Could you check a few things on this model? Use its own coordinates, in mm. A direction names the side the tool comes from. Give positions to 0.01 mm unless a question says otherwise; leave off trailing zeros. Order: outer loops, then holes, each group sorted by start corner. A loop starts at its lowest first (then second) coordinate and runs counter-clockwise, first axis right, second up. Notation, with made-up numbers: (80.25, -32) - (111.25, -32) arc R18 cw to (111.25, -16) - close; hole circle Ø6 at (33, 29). An arc over 180 degrees is marked (long way). Put each result on its own line as item: value.
from build123d import *

# Parameters (mm, degrees)
PAD_DEPTH    = 1.5
PAD001_DEPTH = 0.9


with BuildPart() as body:
    # Sketch → Pad (new body)
    with BuildSketch(Plane.XY):
        with BuildLine():
            ThreePointArc((92, 56.2709215446), (72.3076923077, 26.7324600061), (92, -2.8060015324))
            ThreePointArc((91.6153846154, -3.7290784554), (92.2692307692, -3.4598476862), (92, -2.8060015324))
            ThreePointArc((91.6153846154, -3.7290784554), (89, -4.8060015324), (90.0769230769, -7.4213861477))
            ThreePointArc((90.0769230769, -7.4213861477), (95.9615384615, -4.9983092247), (93.5384615385, 0.88630616))
            ThreePointArc((93.5384615385, 52.5786138523), (76.3076923077, 26.7324600061), (93.5384615385, 0.88630616))
            ThreePointArc((93.5384615385, 52.5786138523), (95.9615384615, 58.4632292369), (90.0769230769, 60.88630616))
            ThreePointArc((90.0769230769, 60.88630616), (89, 58.2709215446), (91.6153846154, 57.1939984676))
            ThreePointArc((92, 56.2709215446), (92.2692307692, 56.9247676984), (91.6153846154, 57.1939984676))
        make_face()
    extrude(amount=PAD_DEPTH)

    # Sketch001 → Pad001 (join)
    with BuildSketch(Plane.XY):
        with BuildLine():
            ThreePointArc((0, 20), (29.323857539, 21.0437591192), (58.4992960523, 24.1697536209))
            ThreePointArc((58.4992960523, 24.1697536209), (68.0731220762, 28.4157701053), (74.013620455, 37.0411558783))
            ThreePointArc((74.013620455, 37.0411558783), (74.1652431283, 15.9884962371), (87.3639974769, -0.4136484716))
            ThreePointArc((87.3639974769, -0.4136484716), (75.7108888805, 4.2658460628), (63.1588059736, 4.6370922787))
            ThreePointArc((0, 0), (31.664401924, 1.1608311192), (63.1588059736, 4.6370922787))
            Line((0, 20), (0, 0))
        make_face()
        with BuildLine():
            ThreePointArc((8.0757502279, 6.0764743472), (36.8018825362, 7.5909701802), (65.3605544983, 11.0386695272))
            ThreePointArc((65.3605544983, 11.0386695272), (68.7002124728, 15.6044864983), (64.1343955017, 18.9441444728))
            ThreePointArc((7.9242497721, 14.0750396943), (36.1114820384, 15.5611237014), (64.1343955017, 18.9441444728))
            ThreePointArc((7.9242497721, 14.0750396943), (4.0007173264, 10.0000067928), (8.0757502279, 6.0764743472))
        make_face(mode=Mode.SUBTRACT)
    extrude(amount=PAD001_DEPTH)


with BuildPart() as part_mirroring:
    # Part__Mirroring: instance of Body
    add(body.part.mirror(Plane(origin=(0, 0, 0), x_dir=(0, -1, 0), z_dir=(1, 0, 0))))


solid = part_mirroring.part
1) If I drill on line 1 (Z direction, x = -71, y = 29.5); line 2 (Y direction, x = -40.5, z = 0.1); line 3 (Y direction, x = -57, z = 0.35), over which ranges is the centre line in solid material (lowest first)? Write a range as [from, to].
Filled in:
line 1: z = [0, 0.9]
line 2: y = [1.9, 7.93], [15.96, 21.99]
line 3: y = [3.77, 9.83], [17.9, 23.96]
2) Suppose I cut it at B-B, the plane x = -84.5. List the corners of the cut face in (y, z) for me, and give its area (3 significant figures).
Filled in:
outline: (1.2, 0) - (6.94, 0) - (6.94, 1.5) - (1.6, 1.5) - (1.6, 0.9) - (1.2, 0.9) - close; (46.52, 0) - (51.87, 0) - (51.87, 1.5) - (46.52, 1.5) - close
area: 16.4 mm^2
3) We'd pull the mould along X, two halves only. Please class faces 4 (the cylindrical face through (-36.401, 7.556, 0.444)), 5 (the cylindrical face through (-95.92, -5.09, 0.74)), 6 (the cylindrical face through (-76.31, 27.19, 0.74)): pulls with the +X half, pulls with the -X half, needs draft (parallel to the pull), parting line crosses it, or undercut.
Filled in:
face 4: undercut
face 5: parting line crosses it
face 6: pulls with the -X half
4) Which directions (+Z, -Z, +X, -X, +Y, -Y) give clear straight access to the entire face, cutting with the end or side of a thin tool? Please do faces 1 (the cylindrical face through (-31.22, 1.13, 0.44)), 2 (the cylindrical face through (-35.718, 15.527, 0.444)), 3 (the cylindrical face through (-73.535, 35.508, 1.073)).
Filled in:
face 1: +Z, -Z, -Y
face 2: +Z, -Z
face 3: +Z, +X
5) I'm going to push a flat-ended pin straight in: pin 1 (11 mm diameter, centred on x = -43, y = 20.5, fed in from +Z). Where does the tip first touch, or does it pass through?
Filled in:
pin 1: stops at z = 0.9
6) Suppose I cut it at A-A, the plane y = 12. List the corners of the cut face in (x, z) for me.
Filled in:
outline: (-80.5, 0) - (-67.4, 0) - (-67.4, 0.9) - (-75.9, 0.9) - (-75.9, 1.5) - (-80.5, 1.5) - close; (-4.49, 0) - (0, 0) - (0, 0.9) - (-4.49, 0.9) - close
7) Suppose I cut it at D-D, the plane x = -17. List the corners of the cut face in (y, z) for me, and give its area (3 significant figures).
Filled in:
outline: (0.33, 0) - (6.34, 0) - (6.34, 0.9) - (0.33, 0.9) - close; (14.35, 0) - (20.35, 0) - (20.35, 0.9) - (14.35, 0.9) - close
area: 10.8 mm^2
8) Suppose I cut it at C-C, the plane z = 0.3. List the corners of the cut face in (x, y) for me.
Filled in:
outline: (-93.54, 0.89) arc R4.5 ccw to (-90.08, -7.42) arc R2 ccw to (-91.62, -3.73) arc R0.5 cw to (-92, -2.81) arc R32 ccw to (-87.36, -0.41) arc R35.83 cw to (-63.16, 4.64) arc R432.44 ccw to (0, 0) - (0, 20) arc R412.44 cw to (-58.5, 24.17) arc R19.28 cw to (-74.01, 37.04) arc R32 ccw to (-92, 56.27) arc R0.5 cw to (-91.62, 57.19) arc R2 ccw to (-90.08, 60.89) arc R4.5 ccw to (-93.54, 52.58) arc R28 cw to start; hole (-65.36, 11.04) arc R426.44 ccw to (-8.08, 6.08) arc R4 ccw to (-7.92, 14.08) arc R418.44 cw to (-64.13, 18.94) arc R4 ccw to start
